Answer from the drawing. Dimensions are ordinates in mm from the lowest x, y and z of the part. A direction names the side the tool comes from. Round coordinates to 2 decimals unless told otherwise and drop trailing zeros. Write each loop counter-clockwise with the first axis right and the second up, starting at its lowest first coordinate (ties: lowest second). Pieces come first, ordered by that corner, then holes. Notation, with made-up numbers: (49, 19) - (90, 19) arc R18 cw to (90, 38) - close; hole circle Ø5 at (76.5, 89). An arc over 180 degrees is marked (long way). One line per item, written item: value. Start each with the question number.
(1) A cutting plane is placed at D-D, the plane x = 8. Determine the outline of the cut face in (y, z).
(2) A cutting plane is placed at C-C, the plane z = 25.5. Determine the outline of the cut face in (x, y), plus the area to 3 significant figures.
(3) Flat-ended cylindrical pins translate along their axes: pin 1 Ø6 at (x, z) = (13.5, 15) entering from +Y; pin 2 Ø8 at (x, y) = (14, 24) entering from -Z (1 decimal); pin 3 Ø1.5 at (y, z) = (31, 16) entering from +X. Find the tip coordinate at first contact, or state that the pin passes through.
(4) A cutting plane is placed at B-B, the plane y = 12.5. Determine the outline of the cut face in (x, z) (1 decimal).
(5) Find the intervals of material crossed by L1, parallel to X at y = 6.5, z = 30.5; L2, parallel to Z at x = 13, y = 18; L3, parallel to Y at x = 5, z = 21, in increasing order.
(6) A cutting plane is placed at A-A, the plane z = 18.5. Determine the outline of the cut face in (x, y) (1 decimal), plus the area to 3 significant figures.
(7) For the marked faces 1, 2 and 3, determine the directions among +Z, -Z, +X, -X, +Y, -Y from which every point of the face is accessible in a straight line to the end or side of a thin tool.
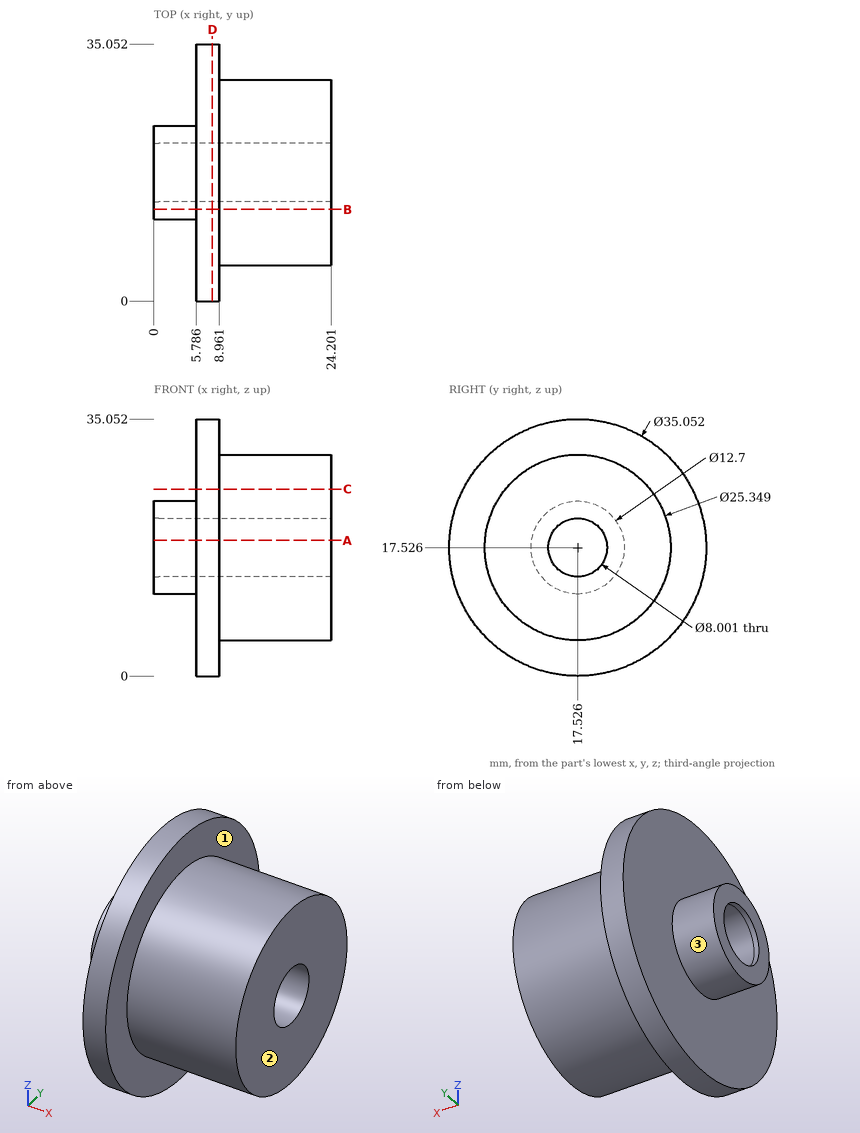
Here are the results:
1. outline: circle Ø35.05 at (17.53, 17.53); hole circle Ø8 at (17.53, 17.53)
2. outline: (5.79, 1.92) - (8.96, 1.92) - (8.96, 7.67) - (24.2, 7.67) - (24.2, 27.38) - (8.96, 27.38) - (8.96, 33.13) - (5.79, 33.13) - close
2. area: 399 mm²
3. pin 1: y = 30.2
3. pin 2: z = 5.1
3. pin 3: x = 8.96
4. outline: (0, 13.6) - (5.8, 13.6) - (5.8, 0.7) - (9, 0.7) - (9, 5.9) - (24.2, 5.9) - (24.2, 29.2) - (9, 29.2) - (9, 34.3) - (5.8, 34.3) - (5.8, 21.4) - (0, 21.4) - close
5. L1: 5.79 to 8.96
5. L2: 4.86 to 13.55, 21.5 to 30.19
5. L3: 12.21 to 15.54, 19.51 to 22.84
6. outline: (0, 11.3) - (5.8, 11.3) - (5.8, 0) - (9, 0) - (9, 4.9) - (24.2, 4.9) - (24.2, 13.6) - (0, 13.6) - close; (0, 21.4) - (24.2, 21.4) - (24.2, 30.2) - (9, 30.2) - (9, 35) - (5.8, 35) - (5.8, 23.8) - (0, 23.8) - close
6. area: 381 mm²
7. face 1: +X
7. face 2: +Z, -Z, +X, +Y, -Y
7. face 3: -X
